```python
from build123d import *

# Parameters (mm, degrees)
SKETCH_R        = 13
SKETCH_R_2      = 8
PAD_DEPTH       = 10
SKETCH001_R     = 4
PAD001_DEPTH    = 35
CHAMFER_SIZE    = 1
CHAMFER001_SIZE = 0.5


with BuildPart() as part:
    # Sketch → Pad (new body)
    with BuildSketch(Plane.XY):
        Circle(SKETCH_R)
        Circle(SKETCH_R_2, mode=Mode.SUBTRACT)
    extrude(amount=PAD_DEPTH)

    # Sketch001 → Pad001 (join)
    with BuildSketch(Plane.XZ.offset(9)):
        with Locations((0, 5)):
            Circle(SKETCH001_R)
    extrude(amount=PAD001_DEPTH)

    # Chamfer
    chamfer_edges = [part.edges().sort_by_distance(p)[0] for p in [
        (-4, -44, 5),
    ]]
    chamfer(chamfer_edges, length=CHAMFER_SIZE)

    # Chamfer001
    chamfer001_edges = [part.edges().sort_by_distance(p)[0] for p in [
        (-8, 0, 10),
    ]]
    chamfer(chamfer001_edges, length=CHAMFER001_SIZE)


solid = part.part
```
Could you check a few things on this model? Use its own coordinates, in mm. A direction names the side the tool comes from. Coordinates: 2 decimals unless noted, no trailing zeros. Loops run counter-clockwise (first coordinate to the right, second up) from the corner with the lowest first, then second, coordinate; pieces in that order, holes last. Notation, with made-up numbers: M 15,42 L 30,42 A28 cw 30,80 Z; hole C -37,64.5 d1. An arc over 180 degrees is marked long. Put each result on its own line as item: value. Start each with the question number.
(1) Suppose I cut it at C-C on y = 0. Please give me the cut outline in (x, z).
(2) I need wall thicknesses on line 1 (Y direction, x = 0, z = 3.25); line 2 (X direction, y = -1, z = 9.5); line 3 (X direction, y = -33, z = 5.25). Which ranges of each line are inside material? Lowest first, please. Write a range as from..to.
(3) Suppose I cut it at D-D on y = -33.5. Please give me the cut outline in (x, z).
(4) For faces 1 (the face through (-0.867, -27.47, 1.095)), 2 (the face through (6, 6, 0)), which set-ups out of +Z, -Z, +X, -X, +Y, -Y let a thin tool reach every point of the face, with its end or its side?
(5) Will these pins go through, and if not, where does the flat tip stop? P1, Ø3, axis at x = 4.5, z = 7.5, coming from the +Y side; P2, Ø9.5, axis at x = 0, y = 0, coming from the +Z side; P3, Ø4, axis at x = -2.5, y = -25.5, coming from the +Z side; P4, Ø1.5, axis at x = -5.5, z = 5.5, coming from the +Y side.
(6) Suppose I cut it at A-A on z = 5. Please give me the cut outline in (x, y), then the cut area to 3 significant figures.
(7) Suppose I cut it at B-B on x = 0. Please give me the cut outline in (y, z), then the cut area to 3 significant figures.
Solutions:
1. outline: M -13,0 L -8,0 L -8,9.5 L -8.5,10 L -13,10 Z; M 8,0 L 13,0 L 13,10 L 8.5,10 L 8,9.5 Z
2. line 1: y = -44..-8, 8..13
2. line 2: x = -12.96..-7.94, 7.94..12.96
2. line 3: x = -3.99..3.99
3. outline: C 0,5 d8
4. face 1: -Y
4. face 2: -Z, +X, -X, +Y, -Y
5. P1: stops at y = 12.65
5. P2: passes through
5. P3: stops at z = 8.97
5. P4: stops at y = 12.1
6. outline: M -4,-43 L -3,-44 L 3,-44 L 4,-43 L 4,-12.37 A13 ccw long -4,-12.37 Z; hole C 0,0 d16
6. area: 579 mm2
7. outline: M -44,2 L -43,1 L -13,1 L -13,0 L -8,0 L -8,9.5 L -8.5,10 L -13,10 L -13,9 L -43,9 L -44,8 Z; M 8,0 L 13,0 L 13,10 L 8.5,10 L 8,9.5 Z
7. area: 347 mm2
